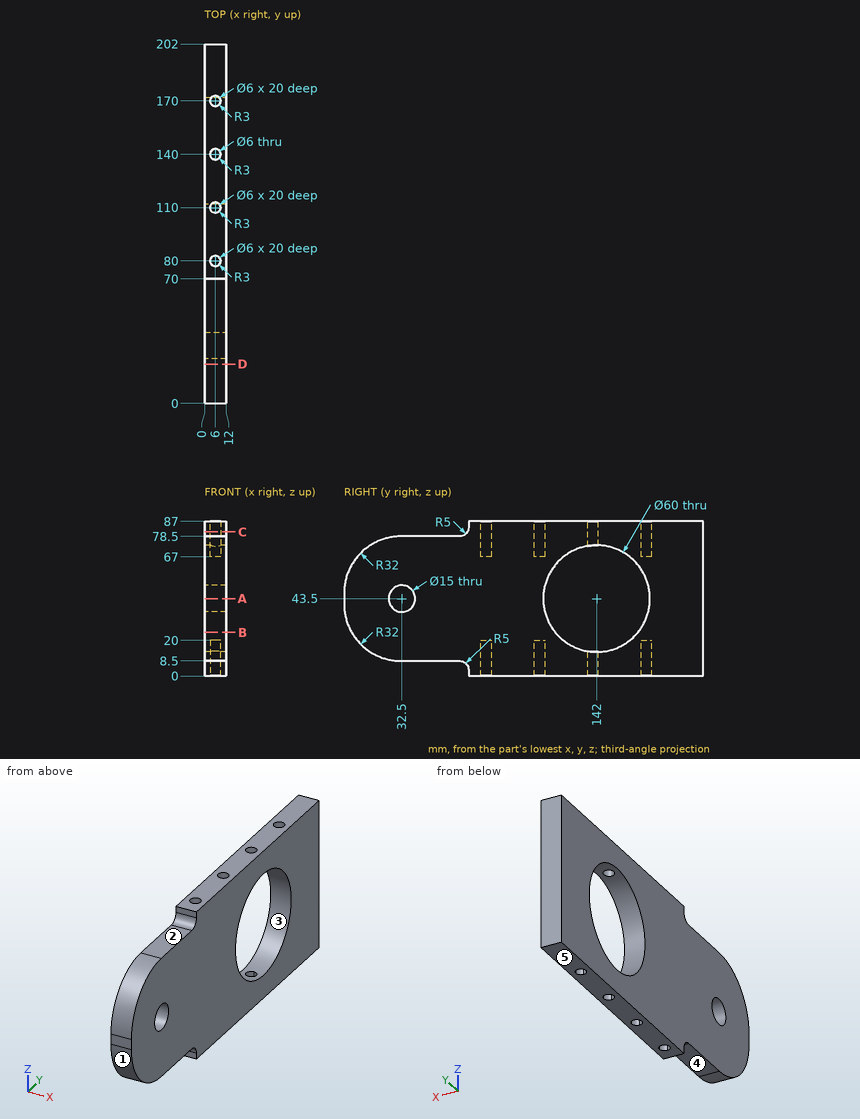
Job drawing, mm, ordinate dimensions from the low corner. One solid piece. A direction names the side the tool comes from. Round coordinates to 2 decimals unless told otherwise and drop trailing zeros. Loops run counter-clockwise (first coordinate to the right, second up) from the corner with the lowest first, then second, coordinate; pieces in that order, holes last. Notation, with made-up numbers: (-3.5, 49.25) -> (28.5, 49.25) arc R17 cw to (28.5, 58.25) -> close; hole circle Ø2 at (46, 54). An arc over 180 degrees is marked (long way). One line per item, written item: value. Start each with the question number.
Q1. Cut at C-C on z = 81. List the corners of the cut face in (x, y), plus the area to 3 significant figures.
Q2. Cut at D-D on y = 22. List the corners of the cut face in (x, z).
Q3. 3-axis set-ups, long thin cutter, end or side, ignore diameter. For the marked faces 4 and 5: which of +Z, -Z, +X, -X, +Y, -Y reach the whole face in a straight line?
Q4. Two-plate mould, pull along Z, no slides. Class the marked faces 1, 2 and 3: released by +Z, released by -Z, zero draft, split by the parting line, or undercut.
Q5. Cut at B-B on z = 24.5. List the corners of the cut face in (x, y), plus the area to 3 significant figures.
Q6. Probe line 1 along Z through (x, y) = (11.75, 33); line 2 along X through (y, z) = (140, 79.25); line 3 along Y through (x, z) = (8.5, 38.5). List the from-to ranges inside material, lowest first.
Q7. Drop flat-ended pins along their axis: pin 1 Ø6 at (x, y) = (2.5, 55) entering from +Z; pin 2 Ø1.8 at (x, y) = (5, 109.5) entering from -Z; pin 3 Ø3 at (x, z) = (3.5, 2.5) entering from -Y. Give the stop position or say it passes through.
Q8. Cut at A-A on z = 43.5. List the corners of the cut face in (x, y).
Computed:
1. outline: (0, 69.33) -> (12, 69.33) -> (12, 202) -> (0, 202) -> close; hole circle Ø6 at (6, 80); hole circle Ø6 at (6, 110); hole circle Ø6 at (6, 140); hole circle Ø6 at (6, 170)
1. area: 1,480 mm²
2. outline: (0, 10.1) -> (12, 10.1) -> (12, 76.9) -> (0, 76.9) -> close
3. face 4: -Z, +X, -X, -Y
3. face 5: -Z, +X, -X, +Y, -Y
4. face 1: released by -Z
4. face 2: released by +Z
4. face 3: undercut
5. outline: (0, 4.29) -> (12, 4.29) -> (12, 118.78) -> (0, 118.78) -> close; (0, 165.22) -> (12, 165.22) -> (12, 202) -> (0, 202) -> close
5. area: 1,820 mm²
6. line 1: 8.5 to 36.02, 50.98 to 78.5
6. line 2: 0 to 3, 9 to 12
6. line 3: 0.06 to 26.91, 38.09 to 112.42, 171.58 to 202
7. pin 1: z = 78.5
7. pin 2: z = 20
7. pin 3: y = 69.97
8. outline: (0, 0) -> (12, 0) -> (12, 25) -> (0, 25) -> close; (0, 40) -> (12, 40) -> (12, 112) -> (0, 112) -> close; (0, 172) -> (12, 172) -> (12, 202) -> (0, 202) -> close
